For this review, take the finished solid that the model builds, in its own axes (mm). Face numbers are marked on the shaded views. Round coordinates to 2 decimals unless told otherwise and drop trailing zeros. Write each loop counter-clockwise with the first axis right and the second up, starting at its lowest first coordinate (ties: lowest second). Pieces come first, ordered by that corner, then holes. Notation, with made-up numbers: (34, 72.25) - (84, 72.25) arc R21 ccw to (84, 87.25) - close; hole circle Ø5 at (34, 23.5). An arc over 180 degrees is marked (long way). One line per item, written item: value. Start each with the question number.
Q1. Clearance check with flat-ended pins moving along their axes: pin 1 Ø6 at (x, y) = (33, 86) entering from -Z; pin 2 Ø3 at (y, z) = (-34.5, -23.5) entering from -X; pin 3 Ø18.5 at (y, z) = (-144, 14) entering from -X; pin 4 Ø24 at (x, z) = (10, -80) entering from +Y. State where each tip first meets the part, or that it passes through.
Q2. Add section C-C on y = -138. Write out the cut boundary in (x, z).
Q3. Add section B-B on z = -8. Write out the cut boundary in (x, y), and give its area (3 significant figures).
Q4. Add section A-A on x = -90. Write out the cut boundary in (y, z), and give its area (3 significant figures).
Q5. Mouldability with a two-part tool opening along Y and no side actions: class the marked faces 1, 2 and 3 as +Y half, -Y half, draft (parallel to the pull), parting line (faces both ways), or undercut.
Q6. Add section D-D on z = -69. Write out the cut boundary in (x, y).
Q7. For probe 1 along Y at (x, z) = (-29, -70); probe 2 along Y at (x, z) = (97, 7); probe 3 along Z at (x, y) = (3.5, 21), list the stretches that pass through material, from the lowest coordinate up.
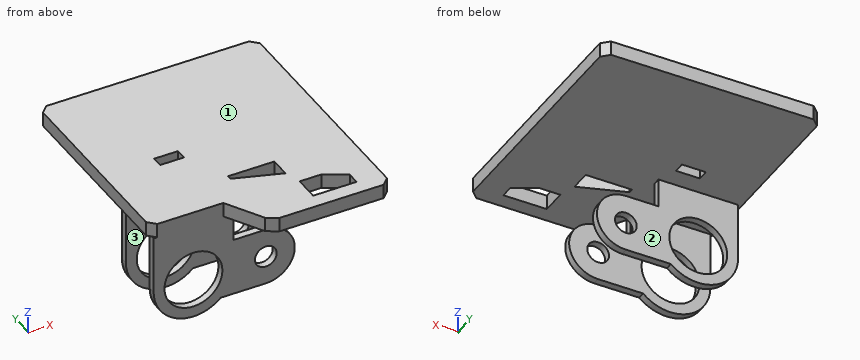
```python
from build123d import *

# Parameters (mm, degrees)
SKETCH2_W           = 33
SKETCH2_H           = 15
BOSS_EXTRUDE1_DEPTH = 20
SKETCH8_R           = 40
SKETCH8_R_2         = 15
BOSS_EXTRUDE3_DEPTH = 10
LPATTERN1_COUNT     = 2
LPATTERN1_PITCH     = 70


with BuildPart() as part:
    # Sketch2 → Boss-Extrude1 (new body)
    with BuildSketch(Plane.XY):
        Polygon((-140, -110), (-48.782097787, -110), (-19.141081636, -161.339745962), (-4.141081636, -170), (140, -170), (150, -160), (150, 160), (140, 170), (-140, 170), (-150, 160), (-150, -100), align=None)
        Polygon((84, -115), (114, -132), (114, -149), (54, -149), (54, -115), align=None, mode=Mode.SUBTRACT)
        Polygon((47, -92), (-17, -70), (-17, -64), (47, -64), align=None, mode=Mode.SUBTRACT)
        with Locations((-61.5, 3.5)):
            Rectangle(SKETCH2_W, SKETCH2_H, mode=Mode.SUBTRACT)
    extrude(amount=BOSS_EXTRUDE1_DEPTH)

    # Sketch8 → Boss-Extrude3 (add)
    with BuildSketch(Plane.XZ.offset(110)):
        with BuildLine():
            Line((-145, 0), (-145, -80))
            ThreePointArc((-145, -80), (-111.780674121, -130.503487353), (-52.250827824, -120))
            Line((-52.250827824, -120), (10, -120))
            ThreePointArc((10, -120), (50, -80), (10, -40))
            Line((10, -40), (-35, -40))
            Line((-35, -40), (-35, 0))
            Line((-35, 0), (-145, 0))
        make_face()
        with Locations((-90, -80)):
            Circle(SKETCH8_R, mode=Mode.SUBTRACT)
        with Locations((10, -80)):
            Circle(SKETCH8_R_2, mode=Mode.SUBTRACT)
    boss_extrude3 = extrude(amount=-BOSS_EXTRUDE3_DEPTH)

    # LPattern1: Boss-Extrude3 ×2
    with Locations(*[(0, i * LPATTERN1_PITCH, 0) for i in range(1, LPATTERN1_COUNT)]):
        add(boss_extrude3)


solid = part.part
```
Result set:
1. pin 1: stops at z = 0
1. pin 2: stops at x = -145
1. pin 3: stops at x = -34.49
1. pin 4: passes through
2. outline: (-32.62, 0) - (54, 0) - (54, 20) - (-32.62, 20) - close; (114, 0) - (150, 0) - (150, 20) - (114, 20) - close
3. outline: (-145, -110) - (-35, -110) - (-35, -100) - (-145, -100) - close; (-145, -40) - (-35, -40) - (-35, -30) - (-145, -30) - close
3. area: 2,200 mm^2
4. outline: (-110, -135) - (-100, -135) - (-100, -120) - (-110, -120) - close; (-110, -40) - (-100, -40) - (-100, 0) - (-40, 0) - (-40, -40) - (-30, -40) - (-30, 0) - (170, 0) - (170, 20) - (-110, 20) - close; (-40, -135) - (-30, -135) - (-30, -120) - (-40, -120) - close
4. area: 6,700 mm^2
5. face 1: draft
5. face 2: +Y half
5. face 3: undercut
6. outline: (-145, -110) - (-128.46, -110) - (-128.46, -100) - (-145, -100) - close; (-145, -40) - (-128.46, -40) - (-128.46, -30) - (-145, -30) - close; (-51.54, -110) - (-0.2, -110) - (-0.2, -100) - (-51.54, -100) - close; (-51.54, -40) - (-0.2, -40) - (-0.2, -30) - (-51.54, -30) - close; (20.2, -110) - (48.46, -110) - (48.46, -100) - (20.2, -100) - close; (20.2, -40) - (48.46, -40) - (48.46, -30) - (20.2, -30) - close
7. probe 1: y = -110 to -100, -40 to -30
7. probe 2: y = -170 to -149, -122.37 to 170
7. probe 3: z = 0 to 20
